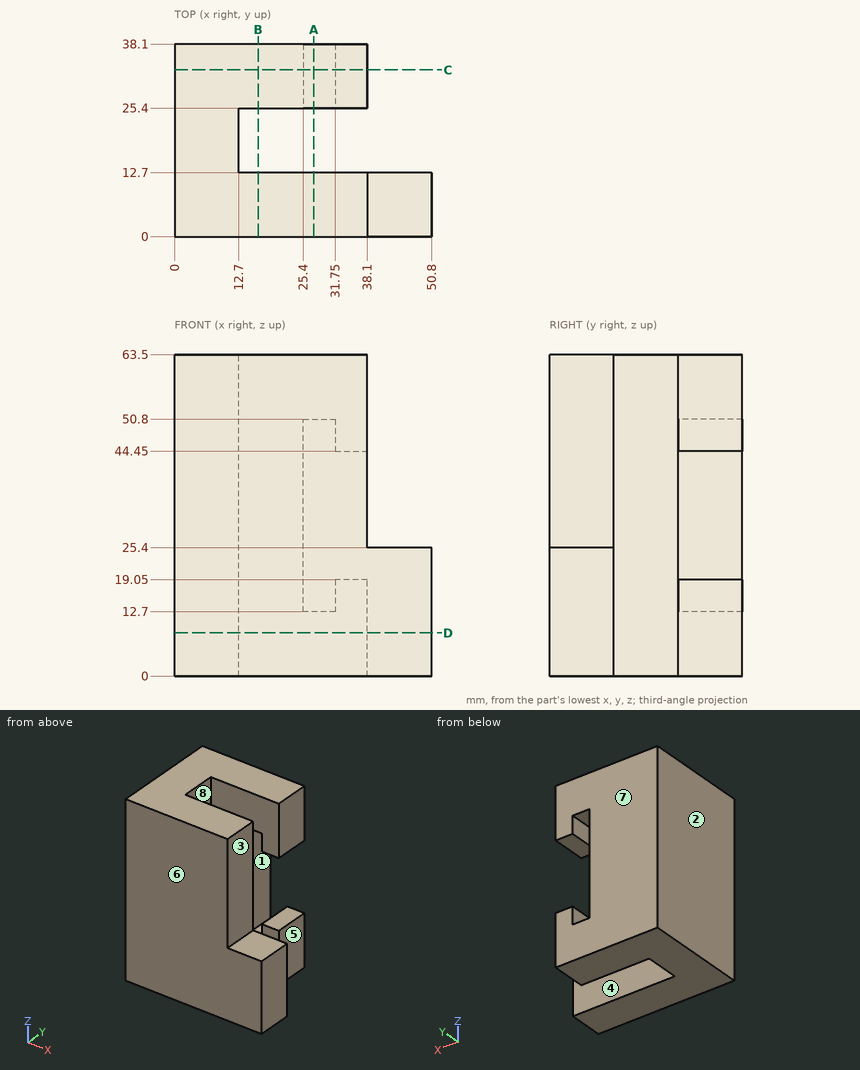
The drawing under review shows one solid part. Ordinate dimensions are in mm from its lowest x, y, z. A direction names the side the tool comes from. Coordinates: 2 decimals unless noted, no trailing zeros. Order: outer loops, then holes, each group sorted by start corner. A loop starts at its lowest first (then second) coordinate and runs counter-clockwise, first axis right, second up. Notation, with made-up numbers: (-32, 27.5) -> (-1, 27.5) arc R28 cw to (-1, 50.5) -> close; hole circle Ø11 at (64, 36.25). An arc over 180 degrees is marked (long way). Answer as CSV lines item,"result".
Q1. We need section B-B (x = 16.5). State the section outline as (y, z) points, plus the area to 3 significant figures.
Model answer:
outline,"(0, 0) -> (12.7, 0) -> (12.7, 63.5) -> (0, 63.5) -> close; (25.4, 0) -> (38.1, 0) -> (38.1, 63.5) -> (25.4, 63.5) -> close"
area,"1,610 mm2"
Q2. We need section A-A (x = 27.5). State the section outline as (y, z) points.
Model answer:
outline,"(0, 0) -> (12.7, 0) -> (12.7, 63.5) -> (0, 63.5) -> close; (25.4, 0) -> (38.1, 0) -> (38.1, 12.7) -> (25.4, 12.7) -> close; (25.4, 50.8) -> (38.1, 50.8) -> (38.1, 63.5) -> (25.4, 63.5) -> close"
Q3. Draft analysis for pull direction Y (two halves, no side actions). For the marked faces 5, 6, 7 and 8, state which applies: released by +Y, released by -Y, zero draft, split by the parting line, or undercut.
Model answer:
face 5,"zero draft"
face 6,"released by -Y"
face 7,"released by +Y"
face 8,"undercut"
Q4. We need section C-C (y = 33). State the section outline as (x, z) points.
Model answer:
outline,"(0, 0) -> (38.1, 0) -> (38.1, 19.05) -> (31.75, 19.05) -> (31.75, 12.7) -> (25.4, 12.7) -> (25.4, 50.8) -> (31.75, 50.8) -> (31.75, 44.45) -> (38.1, 44.45) -> (38.1, 63.5) -> (0, 63.5) -> close"
Q5. Clearance check with flat-ended pins moving along their axes: pin 1 Ø10 at (y, z) = (28.5, 54.5) entering from +X; pin 2 Ø4 at (y, z) = (32, 25.5) entering from +X; pin 3 Ø4 at (x, y) = (47, 7) entering from +Z. State where each tip first meets the part, or that it passes through.
Model answer:
pin 1,"stops at x = 38.1"
pin 2,"stops at x = 25.4"
pin 3,"stops at z = 25.4"
Q6. For the marked faces 1, 2, 3 and 4, list the 3-axis set-ups (+Z, -Z, +X, -X, +Y, -Y) from which the entire face can be reached by the end or side of a thin tool; tool diameter is ignored.
Model answer:
face 1,"+Y"
face 2,"+Z, -Z, -X, +Y, -Y"
face 3,"+Z, +X, +Y, -Y"
face 4,"+Z, -Z, +X"
Q7. Wall thickness on line 1 along Y through (x, z) = (21, 15); line 2 along Z through (x, y) = (32, 30); line 3 along X through (y, z) = (34, 18.5): over which ranges is each line inside the solid? List them lowest first. Write a range as [from, to].
Model answer:
line 1,"y = [0, 12.7], [25.4, 38.1]"
line 2,"z = [0, 19.05], [44.45, 63.5]"
line 3,"x = [0, 25.4], [31.75, 38.1]"
Q8. We need section D-D (z = 8.5). State the section outline as (x, y) points.
Model answer:
outline,"(0, 0) -> (50.8, 0) -> (50.8, 12.7) -> (12.7, 12.7) -> (12.7, 25.4) -> (38.1, 25.4) -> (38.1, 38.1) -> (0, 38.1) -> close"
